The drawing under review shows one solid part. Ordinate dimensions are in mm from its lowest x, y, z. Coordinates: 2 decimals unless noted, no trailing zeros. Order: outer loops, then holes, each group sorted by start corner. A loop starts at its lowest first (then second) coordinate and runs counter-clockwise, first axis right, second up. Notation, with made-up numbers: (-13.5, 39) -> (19.5, 39) arc R23 cw to (19.5, 54) -> close; hole circle Ø6 at (44.5, 62). An arc over 180 degrees is marked (long way). Write item = value, one per line.
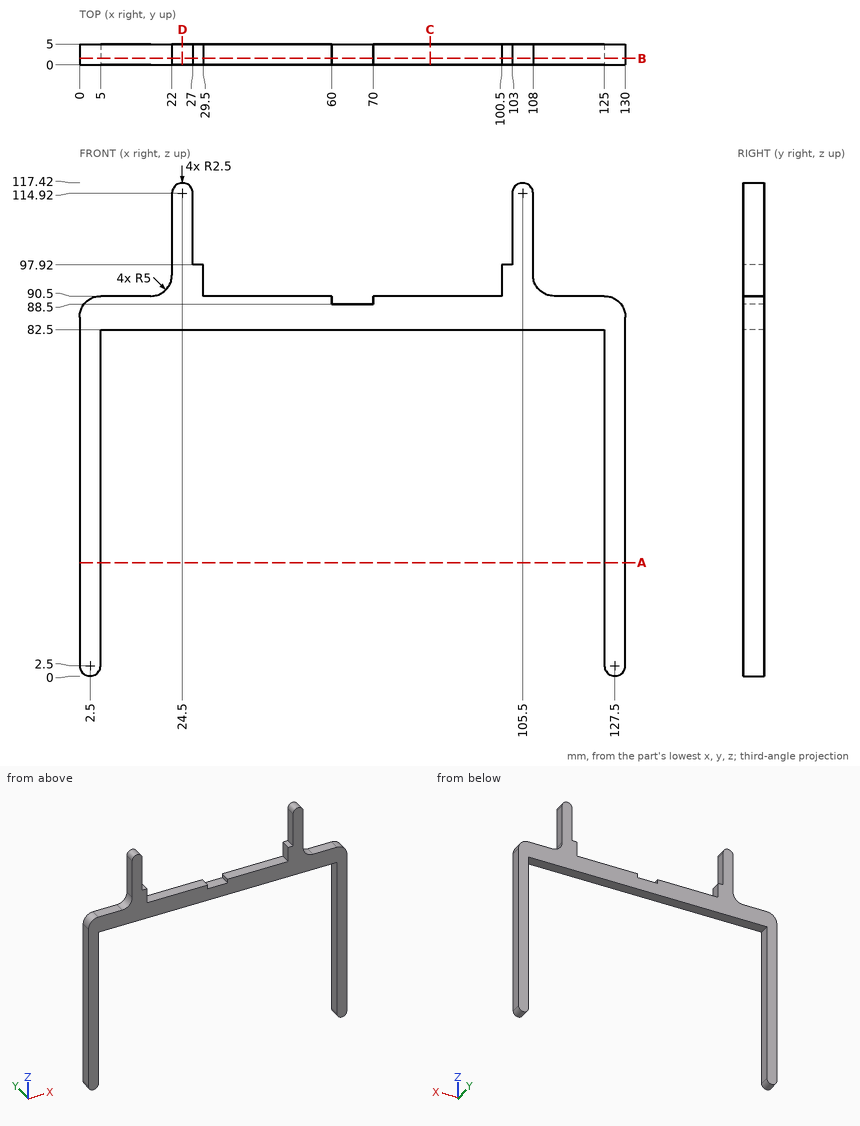
(1) We need section A-A (z = 27). Write out the cut boundary in (x, y).
Report:
outline = (0, 0) -> (5, 0) -> (5, 5) -> (0, 5) -> close; (125, 0) -> (130, 0) -> (130, 5) -> (125, 5) -> close
(2) For L1, parallel to X at y = 2.95, z = 13.5; L2, parallel to X at y = 3.65, z = 98; L3, parallel to Z at x = 11.5, y = 3.55, list the stretches that pass through material, from the lowest coordinate up.
Report:
L1 = 0 to 5, 125 to 130
L2 = 22 to 27, 103 to 108
L3 = 82.5 to 90.5
(3) Insertion check: pin 1 (0.6 mm diameter, centred on y = 2.5, z = 89.5, fed in from -X); pin 2 (4 mm diameter, centred on x = 36, z = 79, fed in from -Y); pin 3 (2.5 mm diameter, centred on y = 2.5, z = 103, fed in from -X); pin 4 (2 mm diameter, centred on y = 3.5, z = 89, fed in from +X). Each pin has a flat end and moves straight along its axis. Give the tip position at first contact, or say it passes through.
Report:
pin_1 = 1.64
pin_2 = through
pin_3 = 22
pin_4 = 129.33
(4) We need section B-B (y = 1.55). Write out the cut boundary in (x, z).
Report:
outline = (0, 2.5) arc R2.5 ccw to (5, 2.5) -> (5, 82.5) -> (125, 82.5) -> (125, 2.5) arc R2.5 ccw to (130, 2.5) -> (130, 85.5) arc R5 ccw to (125, 90.5) -> (113, 90.5) arc R5 cw to (108, 95.5) -> (108, 114.92) arc R2.5 ccw to (103, 114.92) -> (103, 97.92) -> (100.5, 97.92) -> (100.5, 90.5) -> (70, 90.5) -> (70, 88.5) -> (60, 88.5) -> (60, 90.5) -> (29.5, 90.5) -> (29.5, 97.92) -> (27, 97.92) -> (27, 114.92) arc R2.5 ccw to (22, 114.92) -> (22, 95.5) arc R5 cw to (17, 90.5) -> (5, 90.5) arc R5 ccw to (0, 85.5) -> close
(5) We need section D-D (x = 24.5). Write out the cut boundary in (y, z).
Report:
outline = (0, 82.5) -> (5, 82.5) -> (5, 117.42) -> (0, 117.42) -> close
(6) We need section C-C (x = 83.5). Write out the cut boundary in (y, z), and give its area (3 significant figures).
Report:
outline = (0, 82.5) -> (5, 82.5) -> (5, 90.5) -> (0, 90.5) -> close
area = 40.0 mm²
